```python
from build123d import *

# Parameters (mm, degrees)
BOSS_EXTRUDE1_DEPTH    = 3.175
F_10_CLEARANCE_HOLE1_D = 5.1054
FILLET1_R              = 0.635


with BuildPart() as part:
    # Sketch1 → Boss-Extrude1 (new body)
    with BuildSketch(Plane.XY):
        Polygon((15.875, 12.7), (-15.875, 12.7), (-19.05, 9.525), (-19.05, -9.525), (-15.875, -12.7), (15.875, -12.7), (19.05, -9.525), (19.05, 9.525), align=None)
    extrude(amount=BOSS_EXTRUDE1_DEPTH)

    # #10 Clearance Hole1 (through all)
    with Locations(Plane.XY.offset(3.175)):
        with Locations((12.7, 0), (-12.7, 0)):
            Hole(F_10_CLEARANCE_HOLE1_D / 2)

    # Fillet1
    fillet1_edges = [part.edges().sort_by_distance(p)[0] for p in [
        (-17.4625, -11.1125, 3.175),
        (-19.05, 0, 0),
        (-17.4625, 11.1125, 0),
        (0, -12.7, 3.175),
        (17.4625, -11.1125, 3.175),
        (19.05, 0, 3.175),
        (17.4625, 11.1125, 3.175),
        (0, 12.7, 3.175),
        (-10.1473, 0, 3.175),
        (-10.1473, 0, 0),
        (15.2527, 0, 3.175),
        (15.2527, 0, 0),
        (-17.4625, 11.1125, 3.175),
        (-19.05, 0, 3.175),
        (0, 12.7, 0),
        (17.4625, 11.1125, 0),
        (19.05, 0, 0),
        (17.4625, -11.1125, 0),
        (0, -12.7, 0),
        (-17.4625, -11.1125, 0),
    ]]
    fillet(fillet1_edges, radius=FILLET1_R)


solid = part.part
```
Check sheet for the modelled part. Datum: model origin and axes. Units: mm. Give positions to 0.01 mm unless a question says otherwise; leave off trailing zeros. Loops run counter-clockwise (first coordinate to the right, second up) from the corner with the lowest first, then second, coordinate; pieces in that order, holes last. Notation, with made-up numbers: M 38,13 L 71,13 A13 ccw 71,32 Z; hole C -25.5,16 d8. An arc over 180 degrees is marked long. Answer in a Markdown table with one row per item.
1) Thickness scan on line 1 (Y direction, x = 12.7, z = 1.35); line 2 (X direction, y = 1, z = 0.85); line 3 (Y direction, x = -13.5, z = 0.65). Record the ranges inside material, lowest first.
Solutions:
| item | result |
|---|---|
| line 1 | y = -12.7 to -2.55, 2.55 to 12.7 |
| line 2 | x = -19.05 to -15.05, -10.35 to 10.35, 15.05 to 19.05 |
| line 3 | y = -12.7 to -2.42, 2.42 to 12.7 |
2) Cross-section at A-A (x = -12.7). Enter the section's corners in (y, z) (3 decimals).
Solutions:
| item | result |
|---|---|
| outline | M -12.7,0.635 A0.635 ccw -12.065,0 L -3.188,0 A0.635 ccw -2.553,0.635 L -2.553,2.54 A0.635 ccw -3.188,3.175 L -12.065,3.175 A0.635 ccw -12.7,2.54 Z; M 2.553,0.635 A0.635 ccw 3.188,0 L 12.065,0 A0.635 ccw 12.7,0.635 L 12.7,2.54 A0.635 ccw 12.065,3.175 L 3.188,3.175 A0.635 ccw 2.553,2.54 Z |
3) Cross-section at C-C (y = 0). Enter the section's corners in (x, z) (3 decimals), plus the area to 3 significant figures.
Solutions:
| item | result |
|---|---|
| outline | M -19.05,0.635 A0.635 ccw -18.415,0 L -15.888,0 A0.635 ccw -15.253,0.635 L -15.253,2.54 A0.635 ccw -15.888,3.175 L -18.415,3.175 A0.635 ccw -19.05,2.54 Z; M -10.147,0.635 A0.635 ccw -9.512,0 L 9.512,0 A0.635 ccw 10.147,0.635 L 10.147,2.54 A0.635 ccw 9.512,3.175 L -9.512,3.175 A0.635 ccw -10.147,2.54 Z; M 15.253,0.635 A0.635 ccw 15.888,0 L 18.415,0 A0.635 ccw 19.05,0.635 L 19.05,2.54 A0.635 ccw 18.415,3.175 L 15.888,3.175 A0.635 ccw 15.253,2.54 Z |
| area | 87.5 mm^2 |
4) Cross-section at B-B (z = 1.6). Enter the section's corners in (x, y) (3 decimals), plus the area to 3 significant figures.
Solutions:
| item | result |
|---|---|
| outline | M -19.05,-9.525 L -15.875,-12.7 L 15.875,-12.7 L 19.05,-9.525 L 19.05,9.525 L 15.875,12.7 L -15.875,12.7 L -19.05,9.525 Z; hole C -12.7,0 d5.105; hole C 12.7,0 d5.105 |
| area | 907 mm^2 |
5) Mould release check, pull along Y, two halves, no side actions. Record for faces 1 (the face through (17.485, 11.09, 1.574)), 2 (the face through (10.265, 0.767, 1.574)), 3 (the face through (0, 0, 0)): released by +Y, released by -Y, zero draft, split by the parting line, or undercut.
Solutions:
| item | result |
|---|---|
| face 1 | released by +Y |
| face 2 | undercut |
| face 3 | zero draft |
6) Depth check by flat-ended pin: pin 1 (6 mm diameter, centred on x = -12.7, y = 0, fed in from +Z). Enter the tip coordinate at first touch or a pass-through.
Solutions:
| item | result |
|---|---|
| pin 1 | stops at z = 3.15 |
